from build123d import *

# Parameters (mm, degrees)
BOSS_EXTRUDE1_DEPTH = 6.35
SKETCH2_R           = 1.5
SKETCH2_R_2         = 1.35
CUT_EXTRUDE1_DEPTH  = 80.311553383
CUT_EXTRUDE3_DEPTH  = 80.311553383
SKETCH7_W           = 6.35
SKETCH7_H           = 13
BOSS_EXTRUDE3_DEPTH = 6.35


with BuildPart() as part:
    # Sketch1 → Boss-Extrude1 (new body)
    with BuildSketch(Plane.XY):
        with BuildLine():
            Line((-25, 0), (-25, -75))
            Line((-25, -75), (25, -75))
            Line((25, -75), (25, 0))
            ThreePointArc((25, 0), (0, 25), (-25, 0))
        make_face()
    extrude(amount=BOSS_EXTRUDE1_DEPTH)

    # Sketch2 → Cut-Extrude1 (cut, through all)
    with BuildSketch(Plane.XY.offset(6.35)):
        Circle(SKETCH2_R)
        with Locations((0, 10)):
            Circle(SKETCH2_R_2)
        with Locations((0, -10)):
            Circle(SKETCH2_R_2)
    extrude(amount=-CUT_EXTRUDE1_DEPTH, mode=Mode.SUBTRACT)

    # Sketch6 → Cut-Extrude3 (cut, through all)
    with BuildSketch(Plane.XY.offset(6.35)):
        Polygon((-12.3, -67.54), (-16.999, -67.54), (-16.999, -70.4991), (-20.301, -70.4991), (-20.301, -67.54), (-25, -67.54), (-25, -62.46), (-20.301, -62.46), (-20.301, -59.5009), (-16.999, -59.5009), (-16.999, -62.46), (-12.3, -62.46), align=None)
        Polygon((-12.3, -37.54), (-16.999, -37.54), (-16.999, -40.4991), (-20.301, -40.4991), (-20.301, -37.54), (-25, -37.54), (-25, -32.46), (-20.301, -32.46), (-20.301, -29.5009), (-16.999, -29.5009), (-16.999, -32.46), (-12.3, -32.46), align=None)
    extrude(amount=-CUT_EXTRUDE3_DEPTH, mode=Mode.SUBTRACT)

    # Sketch7 → Boss-Extrude3 (add)
    with BuildSketch(Plane.XY.offset(6.35)):
        with Locations((-28.175, -50)):
            Rectangle(SKETCH7_W, SKETCH7_H)
    extrude(amount=-BOSS_EXTRUDE3_DEPTH)


solid = part.part
Here's how the part is built. I have some questions about the finished solid (model axes, mm). A direction names the side the tool comes from. Round coordinates to 2 decimals unless told otherwise and drop trailing zeros. Write each loop counter-clockwise with the first axis right and the second up, starting at its lowest first coordinate (ties: lowest second). Pieces come first, ordered by that corner, then holes.
1. For faces 1 (the flat face through (-15, -37.54, 3)), 2 (the flat face through (-25, -59, 3)), 3 (the flat face through (-25, -40, 3)), 4 (the flat face through (-19, -59.501, 3)), 5 (the flat face through (25, -38, 3)), which set-ups out of +Z, -Z, +X, -X, +Y, -Y let a thin tool reach every point of the face, with its end or its side?
2. I need wall thicknesses on L1, parallel to Y at x = 0, z = 2.5; L2, parallel to Y at x = -22, z = 2.75; L3, parallel to X at y = -62, z = 1.25. Which ranges of each line are inside material? Lowest first, please.
3. Suppose I cut it at A-A (x = 0). List the corners of the cut face in (y, z) for me, and give its area (3 significant figures).
4. Will these pins go through, and if not, where does the flat tip stop? pin 1 Ø3 at (x, z) = (-29.5, 4.5) entering from -Y; pin 2 Ø1.7 at (x, z) = (-18.5, 2.5) entering from +Y; pin 3 Ø1.5 at (y, z) = (-30.5, 2.5) entering from -X.
5. If we mould it in two halves opening along Y, with no side actions, what happens to faces 6 (the flat face through (-28, -56.5, 3)), 7 (the flat face through (-19, -40.499, 3)), 8 (the flat face through (-25, -16, 3))? For each: released by +Y, released by -Y, zero draft, split by the parting line, or undercut.
6. Suppose I cut it at D-D (y = 10). List the corners of the cut face in (x, z) for me, and give its area (3 significant figures).
7. Suppose I cut it at B-B (y = -10). List the corners of the cut face in (x, z) for me.
8. Suppose I cut it at C-C (z = 2.5). State how many separate pieces and enclosed holes the cut face has, and give its area (3 significant figures).
Answer sheet:
1. face 1: +Z, -Z, -X
1. face 2: +Z, -Z, -X, -Y
1. face 3: +Z, -Z, -X, +Y
1. face 4: +Z, -Z
1. face 5: +Z, -Z, +X, +Y, -Y
2. L1: y = -75 to -11.35, -8.65 to -1.5, 1.5 to 8.65, 11.35 to 25
2. L2: y = -75 to -67.54, -62.46 to -37.54, -32.46 to 11.87
2. L3: x = -25 to -20.3, -17 to 25
3. outline: (-75, 0) - (-11.35, 0) - (-11.35, 6.35) - (-75, 6.35) - close; (-8.65, 0) - (-1.5, 0) - (-1.5, 6.35) - (-8.65, 6.35) - close; (1.5, 0) - (8.65, 0) - (8.65, 6.35) - (1.5, 6.35) - close; (11.35, 0) - (25, 0) - (25, 6.35) - (11.35, 6.35) - close
3. area: 582 mm2
4. pin 1: stops at y = -56.5
4. pin 2: stops at y = 17.71
4. pin 3: stops at x = -25
5. face 6: released by -Y
5. face 7: undercut
5. face 8: zero draft
6. outline: (-22.91, 0) - (-1.35, 0) - (-1.35, 6.35) - (-22.91, 6.35) - close; (1.35, 0) - (22.91, 0) - (22.91, 6.35) - (1.35, 6.35) - close
6. area: 274 mm2
7. outline: (-25, 0) - (-1.35, 0) - (-1.35, 6.35) - (-25, 6.35) - close; (1.35, 0) - (25, 0) - (25, 6.35) - (1.35, 6.35) - close
8. separate pieces: 1
8. enclosed holes: 3
8. area: 4,630 mm2
